from build123d import *

# Parameters (mm, degrees)
SKETCH1_W           = 200
SKETCH1_H           = 30
BOSS_EXTRUDE1_DEPTH = 10
SKETCH2_R           = 2.1
CUT_EXTRUDE1_DEPTH  = 11
SKETCH3_R           = 3.1
CUT_EXTRUDE2_DEPTH  = 11
LPATTERN1_COUNT     = 6
LPATTERN1_PITCH     = 15
FILLET1_R           = 5


with BuildPart() as part:
    # Sketch1 → Boss-Extrude1 (new body)
    with BuildSketch(Plane(origin=(0, 0, 0), x_dir=(1, 0, 0), z_dir=(0, 1, 0))):
        Rectangle(SKETCH1_W, SKETCH1_H)
    extrude(amount=BOSS_EXTRUDE1_DEPTH)

    # Sketch2 → Cut-Extrude1 (cut, through all)
    with BuildSketch(Plane(origin=(0, 10, 0), x_dir=(1, 0, 0), z_dir=(0, 1, 0))):
        with Locations((85, 0)):
            Circle(SKETCH2_R)
        with Locations((75, 0)):
            Circle(SKETCH2_R)
    extrude(amount=-CUT_EXTRUDE1_DEPTH, mode=Mode.SUBTRACT)

    # Sketch3 → Cut-Extrude2 (cut, through all)
    with BuildSketch(Plane(origin=(0, 10, 0), x_dir=(1, 0, 0), z_dir=(0, 1, 0))):
        with Locations((-85, 0)):
            Circle(SKETCH3_R)
    cut_extrude2 = extrude(amount=-CUT_EXTRUDE2_DEPTH, mode=Mode.SUBTRACT)

    # LPattern1: Cut-Extrude2 ×6
    with Locations(*[(i * LPATTERN1_PITCH, 0, 0) for i in range(1, LPATTERN1_COUNT)]):
        add(cut_extrude2, mode=Mode.SUBTRACT)

    # Fillet1
    fillet1_edges = [part.edges().sort_by_distance(p)[0] for p in [
        (-100, 5, -15),
        (100, 5, -15),
        (100, 5, 15),
        (-100, 5, 15),
    ]]
    fillet(fillet1_edges, radius=FILLET1_R)


solid = part.part
Work out the finished part from the listing and answer in its coordinate system (mm). Give positions to 0.01 mm unless a question says otherwise; leave off trailing zeros. Order: outer loops, then holes, each group sorted by start corner. A loop starts at its lowest first (then second) coordinate and runs counter-clockwise, first axis right, second up. Notation, with made-up numbers: (73.25, 13.5) -> (130.25, 13.5) arc R34 ccw to (130.25, 46.5) -> close; hole circle Ø10 at (-0.75, 22). An arc over 180 degrees is marked (long way). One line per item, written item: value.
Item 1: Determine the mould class of faces 1 (the cylindrical face through (-99, 5, 13)), 2 (the cylindrical face through (98, 5, 14)), 3 (the cylindrical face through (72.9, 5.07, -0.09)) for opening direction X: released by +X, released by -X, zero draft, split by the parting line, or undercut.
Answer sheet:
face 1: released by -X
face 2: released by +X
face 3: undercut
Item 2: Straight lines are drawn through the part: probe 1 along Z at (x, y) = (75, 3); probe 2 along Z at (x, y) = (-55, 5); probe 3 along X at (y, z) = (3.75, 12). For each, find the intervals that lie inside material, in ascending order.
Answer sheet:
probe 1: -15 to -2.1, 2.1 to 15
probe 2: -15 to -3.1, 3.1 to 15
probe 3: -99.58 to 99.58
Item 3: Find section A-A, the plane x = -25. Give the vertices of the cut face in (y, z), plus the area to 3 significant figures.
Answer sheet:
outline: (0, -15) -> (10, -15) -> (10, -3.1) -> (0, -3.1) -> close; (0, 3.1) -> (10, 3.1) -> (10, 15) -> (0, 15) -> close
area: 238 mm²
Item 4: Find section D-D, the plane x = 85. Give the vertices of the cut face in (y, z).
Answer sheet:
outline: (0, -15) -> (10, -15) -> (10, -2.1) -> (0, -2.1) -> close; (0, 2.1) -> (10, 2.1) -> (10, 15) -> (0, 15) -> close
Item 5: Find section B-B, the plane y = 8.5. State how many separate pieces and enclosed holes the cut face has, plus the area to 3 significant figures.
Answer sheet:
separate pieces: 1
enclosed holes: 8
area: 5,770 mm²
